Can you work these out from the drawing? Everything is in mm from the part's minimum corner. A direction names the side the tool comes from. Coordinates: 2 decimals unless noted, no trailing zeros. Order: outer loops, then holes, each group sorted by start corner. A loop starts at its lowest first (then second) coordinate and runs counter-clockwise, first axis right, second up. Notation, with made-up numbers: (41.25, 67.5) - (61.25, 67.5) arc R16 cw to (61.25, 85.5) - close; hole circle Ø7 at (14.5, 66). An arc over 180 degrees is marked (long way). Use CSV: the item, a comma, the result in double quotes. Start each with the question number.
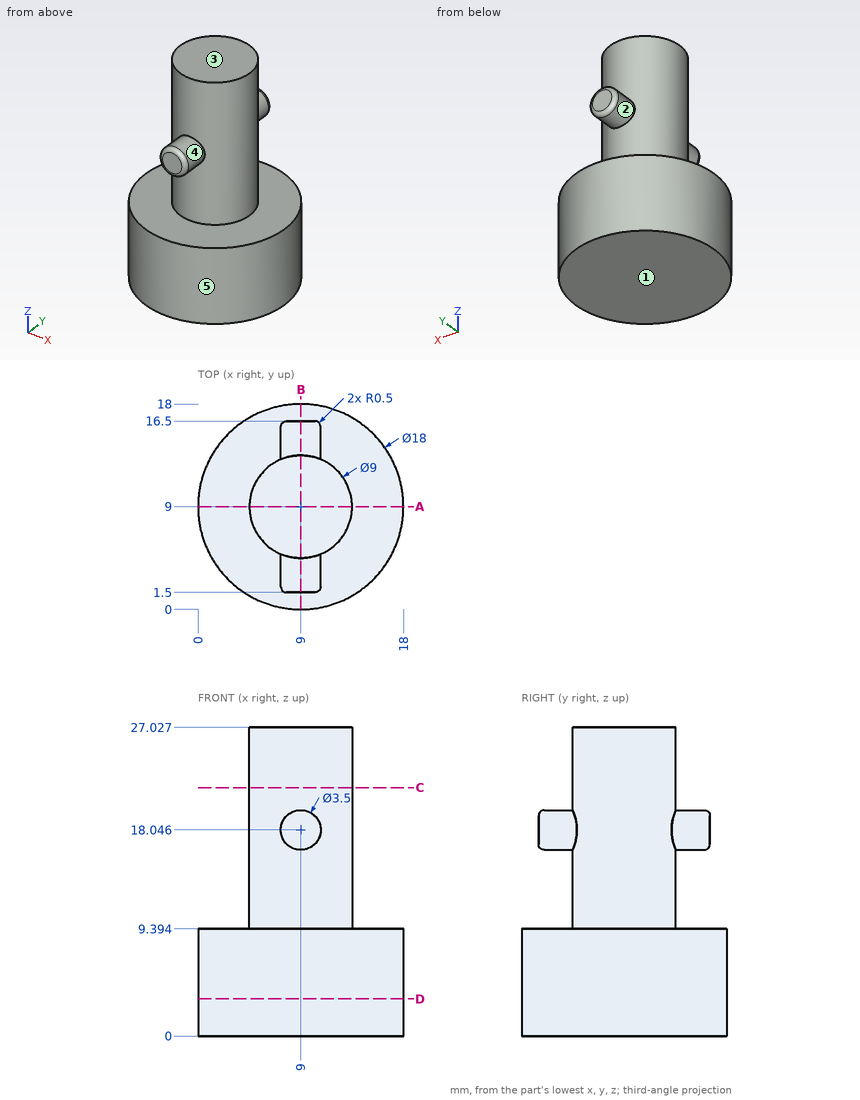
Item 1: Please list where these lines run through material, in increasing order: line 1 along Z through (x, y) = (4.5, 5.5) (1 decimal); line 2 along Y through (x, z) = (9.75, 17); line 3 along Z through (x, y) = (10, 4) (1 decimal). Write a range as from..to.
Item 2: Suppose I cut it at B-B on x = 9. Write out the boundary of the cut face in (y, z) (1 decimal).
Item 3: Suppose I cut it at D-D on z = 3.25. Write out the boundary of the cut face in (x, y).
Item 4: We'd pull the mould along Z, two halves only. Please class the marked faces 3, 4 and 5: released by +Z, released by -Z, zero draft, split by the parting line, or undercut.
Item 5: Suppose I cut it at C-C on z = 21.75. Write out the boundary of the cut face in (x, y).
Item 6: For the marked faces 1 and 2, which set-ups out of +Z, -Z, +X, -X, +Y, -Y let a thin tool reach every point of the face, with its end or its side?
Item 7: For pin 1 Ø3 at (x, z) = (5, 5) entering from -Y (1 decimal); pin 2 Ø10 at (y, z) = (3, 10.5) entering from -X; pin 3 Ø2 at (x, z) = (8.5, 18.5) entering from +Y; pin 4 Ø10 at (x, y) = (11, 14.5) entering from +Z, each with a flat end and sliding along its axis, tell me the tip position at first contact or that it passes through.
Item 8: Suppose I cut it at A-A on y = 9. Write out the boundary of the cut face in (x, z) (1 decimal), then the cut area to 3 significant figures.
Here are the results:
1,line 1,"0..9.4"
1,line 2,"1.5..16.5"
1,line 3,"0..9.4, 16.6..19.5"
2,outline,"(0, 0) - (18, 0) - (18, 9.4) - (13.5, 9.4) - (13.5, 16.3) - (16, 16.3) arc R0.5 ccw to (16.5, 16.8) - (16.5, 19.3) arc R0.5 ccw to (16, 19.8) - (13.5, 19.8) - (13.5, 27) - (4.5, 27) - (4.5, 19.8) - (2, 19.8) arc R0.5 ccw to (1.5, 19.3) - (1.5, 16.8) arc R0.5 ccw to (2, 16.3) - (4.5, 16.3) - (4.5, 9.4) - (0, 9.4) - close"
3,outline,"circle Ø18 at (9, 9)"
4,face 3,"released by +Z"
4,face 4,"undercut"
4,face 5,"zero draft"
5,outline,"circle Ø9 at (9, 9)"
6,face 1,"-Z, +X, -X, +Y, -Y"
6,face 2,"+Y"
7,pin 1,"y = 0.4"
7,pin 2,"x = 0.07"
7,pin 3,"y = 16.5"
7,pin 4,"z = 27.03"
8,outline,"(0, 0) - (18, 0) - (18, 9.4) - (13.5, 9.4) - (13.5, 27) - (4.5, 27) - (4.5, 9.4) - (0, 9.4) - close"
8,area,"328 mm^2"
